CAD build for the part. Positions are in the model's coordinates, mm. A direction names the side the tool comes from. Round coordinates to 2 decimals unless told otherwise and drop trailing zeros. Loops run counter-clockwise (first coordinate to the right, second up) from the corner with the lowest first, then second, coordinate; pieces in that order, holes last.
from build123d import *

# Parameters (mm, degrees)
F0_W          = 36
F0_H          = 20
F1_DEPTH      = 3.5
F3_DEPTH      = 1
F4_W          = 4
F4_H          = 20
F4_W_2        = 8
F5_DEPTH      = 10
F6_R          = 2.5
F7_DEPTH      = 20.001
F8_R          = 5
F9_R          = 3
F10_T4_DEPTH  = 20
F10_T10_DEPTH = 20
F10_T16_DEPTH = 20
F10_T23_DEPTH = 20
F10_T29_DEPTH = 20
F10_T35_DEPTH = 20
F10_T41_DEPTH = 20
F10_T47_DEPTH = 20
F10_T54_DEPTH = 20
F10_T60_DEPTH = 20


# Not quite as in the source:
# - a fillet or chamfer that OpenCascade refuses, or shapes differently, is made with other operations: its cross-section is extruded or revolved along the edge and cut away or added


with BuildPart() as f1:
    # F0 (on Top) → F1 (new body)
    with BuildSketch(Plane.XY):
        Rectangle(F0_W, F0_H)
        with BuildLine():
            ThreePointArc((3.15, 0), (0, -3.15), (-3.15, 0))
            ThreePointArc((-3.15, 0), (0, 3.15), (3.15, 0))
        make_face(mode=Mode.SUBTRACT)
    extrude(amount=F1_DEPTH)

    # F2 (on face) → F3 (cut)
    with BuildSketch(Plane.XY.offset(3.5)):
        with BuildLine():
            Line((-1.3416407865, 2.85), (-8.05, 2.85))
            Line((-8.05, 2.85), (-8.05, -2.85))
            Line((-8.05, -2.85), (-1.3416407865, -2.85))
            ThreePointArc((-1.3416407865, -2.85), (-3.15, 0), (-1.3416407865, 2.85))
        make_face()
        with BuildLine():
            Line((1.3416407865, 2.85), (-1.3416407865, 2.85))
            ThreePointArc((-1.3416407865, 2.85), (-3.15, 0), (-1.3416407865, -2.85))
            Line((-1.3416407865, -2.85), (1.3416407865, -2.85))
            ThreePointArc((1.3416407865, -2.85), (2.6597620643, -1.6876509595), (3.15, 0))
            ThreePointArc((3.15, 0), (2.6597620643, 1.6876509595), (1.3416407865, 2.85))
        make_face()
        with BuildLine():
            Line((8.05, 2.85), (1.3416407865, 2.85))
            ThreePointArc((1.3416407865, 2.85), (2.6597620643, 1.6876509595), (3.15, 0))
            ThreePointArc((3.15, 0), (2.6597620643, -1.6876509595), (1.3416407865, -2.85))
            Line((1.3416407865, -2.85), (8.05, -2.85))
            Line((8.05, -2.85), (8.05, 2.85))
        make_face()
    extrude(amount=-F3_DEPTH, mode=Mode.SUBTRACT)

    # F4 (on Top) → F5 (join)
    with BuildSketch(Plane.XY):
        with Locations((20, 0)):
            Rectangle(F4_W, F4_H)
        with Locations((14, 0)):
            Rectangle(F4_W_2, F4_H)
        with Locations((-14, 0)):
            Rectangle(F4_W_2, F4_H)
        with Locations((-20, 0)):
            Rectangle(F4_W, F4_H)
    extrude(amount=F5_DEPTH)

    # F6 (on face) → F7 (cut, through all)
    with BuildSketch(Plane.XZ.offset(10)):
        with Locations((-16.25, 4.5)):
            Circle(F6_R)
        with BuildLine():
            ThreePointArc((18.75, 4.5), (16.25, 7), (13.75, 4.5))
            ThreePointArc((13.75, 4.5), (16.25, 2), (18.75, 4.5))
        make_face()
    extrude(amount=-F7_DEPTH, mode=Mode.SUBTRACT)

    # F8
    f8_edges = [f1.edges().sort_by_distance(p)[0] for p in [
        (-22, 0, 10),
        (-10, 0, 10),
        (10, 0, 10),
        (22, 0, 10),
    ]]
    fillet(f8_edges, radius=F8_R)

    # F9
    f9_edges = [f1.edges().sort_by_distance(p)[0] for p in [
        (-22, 0, 0),
        (22, 0, 0),
    ]]
    fillet(f9_edges, radius=F9_R)

    # F10: fillet of radius 2.5 on 2 edges, made by hand


with BuildPart() as f10_tool2:
    # F10_s3 → F10_t4 (new body)
    with BuildSketch(Plane.XZ.offset(10)):
        with BuildLine():
            ThreePointArc((10.0446437509, 5.6666666667), (9.2126670979, 4.1180683682), (7.5669656263, 3.5))
            Line((7.5669656263, 3.5), (7.5669656263, 3.25))
            Line((7.5669656263, 3.25), (10, 3.25))
            Line((10, 3.25), (10.25, 3.5))
            ThreePointArc((10.25, 3.5), (10.25, 5), (10.2924115633, 5.6333333333))
            Line((10.2924115633, 5.6333333333), (10.0446437509, 5.6666666667))
        make_face()
    extrude(amount=-F10_T4_DEPTH)

    split(bisect_by=Plane.YZ.offset(8.05), keep=Keep.TOP)

    split(bisect_by=Plane.XZ.offset(2.85), keep=Keep.TOP)


with BuildPart() as f1_1:
    add(f1.part)

    # F10_t1: union F10_tool2
    add(f10_tool2.part)


with BuildPart() as f10_tool8:
    # F10_s9 → F10_t10 (new body)
    with BuildSketch(Plane.XZ.offset(10)):
        with BuildLine():
            ThreePointArc((10.0446437509, 5.6666666667), (9.2126670979, 4.1180683682), (7.5669656263, 3.5))
            Line((7.5669656263, 3.5), (7.5669656263, 3.25))
            Line((7.5669656263, 3.25), (10, 3.25))
            Line((10, 3.25), (10.25, 3.5))
            ThreePointArc((10.25, 3.5), (10.25, 5), (10.2924115633, 5.6333333333))
            Line((10.2924115633, 5.6333333333), (10.0446437509, 5.6666666667))
        make_face()
    extrude(amount=-F10_T10_DEPTH)

    split(bisect_by=Plane.YZ.offset(8.05), keep=Keep.BOTTOM)

    split(bisect_by=Plane.XZ.offset(2.85), keep=Keep.TOP)


with BuildPart() as f1_2:
    add(f1_1.part)

    # F10_t7: union F10_tool8
    add(f10_tool8.part)


with BuildPart() as f10_tool14:
    # F10_s15 → F10_t16 (new body)
    with BuildSketch(Plane.XZ.offset(10)):
        with BuildLine():
            ThreePointArc((10.0446437509, 5.6666666667), (9.2126670979, 4.1180683682), (7.5669656263, 3.5))
            Line((7.5669656263, 3.5), (7.5669656263, 3.25))
            Line((7.5669656263, 3.25), (10, 3.25))
            Line((10, 3.25), (10.25, 3.5))
            ThreePointArc((10.25, 3.5), (10.25, 5), (10.2924115633, 5.6333333333))
            Line((10.2924115633, 5.6333333333), (10.0446437509, 5.6666666667))
        make_face()
    extrude(amount=-F10_T16_DEPTH)

    split(bisect_by=Plane.XZ.offset(-2.85), keep=Keep.TOP)

    split(bisect_by=Plane.YZ.offset(8.05), keep=Keep.TOP)

    split(bisect_by=Plane.XZ.offset(2.85), keep=Keep.BOTTOM)


with BuildPart() as f1_3:
    add(f1_2.part)

    # F10_t13: union F10_tool14
    add(f10_tool14.part)


with BuildPart() as f10_tool21:
    # F10_s22 → F10_t23 (new body)
    with BuildSketch(Plane.XZ.offset(10)):
        with BuildLine():
            ThreePointArc((10.0446437509, 5.6666666667), (9.2126670979, 4.1180683682), (7.5669656263, 3.5))
            Line((7.5669656263, 3.5), (7.5669656263, 3.25))
            Line((7.5669656263, 3.25), (10, 3.25))
            Line((10, 3.25), (10.25, 3.5))
            ThreePointArc((10.25, 3.5), (10.25, 5), (10.2924115633, 5.6333333333))
            Line((10.2924115633, 5.6333333333), (10.0446437509, 5.6666666667))
        make_face()
    extrude(amount=-F10_T23_DEPTH)

    split(bisect_by=Plane.XZ.offset(-2.85), keep=Keep.BOTTOM)

    split(bisect_by=Plane.YZ.offset(8.05), keep=Keep.TOP)


with BuildPart() as f1_4:
    add(f1_3.part)

    # F10_t20: union F10_tool21
    add(f10_tool21.part)


with BuildPart() as f10_tool27:
    # F10_s28 → F10_t29 (new body)
    with BuildSketch(Plane.XZ.offset(10)):
        with BuildLine():
            ThreePointArc((10.0446437509, 5.6666666667), (9.2126670979, 4.1180683682), (7.5669656263, 3.5))
            Line((7.5669656263, 3.5), (7.5669656263, 3.25))
            Line((7.5669656263, 3.25), (10, 3.25))
            Line((10, 3.25), (10.25, 3.5))
            ThreePointArc((10.25, 3.5), (10.25, 5), (10.2924115633, 5.6333333333))
            Line((10.2924115633, 5.6333333333), (10.0446437509, 5.6666666667))
        make_face()
    extrude(amount=-F10_T29_DEPTH)

    split(bisect_by=Plane.XZ.offset(-2.85), keep=Keep.BOTTOM)

    split(bisect_by=Plane.YZ.offset(8.05), keep=Keep.BOTTOM)


with BuildPart() as f1_5:
    add(f1_4.part)

    # F10_t26: union F10_tool27
    add(f10_tool27.part)


with BuildPart() as f10_tool33:
    # F10_s34 → F10_t35 (new body)
    with BuildSketch(Plane.XZ.offset(-10)):
        with BuildLine():
            ThreePointArc((-7.5669656263, 3.5), (-9.2126670979, 4.1180683682), (-10.0446437509, 5.6666666667))
            Line((-10.0446437509, 5.6666666667), (-10.2924115633, 5.6333333333))
            ThreePointArc((-10.2924115633, 5.6333333333), (-10.25, 5), (-10.25, 3.5))
            Line((-10.25, 3.5), (-10, 3.25))
            Line((-10, 3.25), (-7.5669656263, 3.25))
            Line((-7.5669656263, 3.25), (-7.5669656263, 3.5))
        make_face()
    extrude(amount=F10_T35_DEPTH)

    split(bisect_by=Plane.XZ.offset(-2.85), keep=Keep.BOTTOM)

    split(bisect_by=Plane.YZ.offset(-8.05), keep=Keep.TOP)


with BuildPart() as f1_6:
    add(f1_5.part)

    # F10_t32: union F10_tool33
    add(f10_tool33.part)


with BuildPart() as f10_tool39:
    # F10_s40 → F10_t41 (new body)
    with BuildSketch(Plane.XZ.offset(-10)):
        with BuildLine():
            ThreePointArc((-7.5669656263, 3.5), (-9.2126670979, 4.1180683682), (-10.0446437509, 5.6666666667))
            Line((-10.0446437509, 5.6666666667), (-10.2924115633, 5.6333333333))
            ThreePointArc((-10.2924115633, 5.6333333333), (-10.25, 5), (-10.25, 3.5))
            Line((-10.25, 3.5), (-10, 3.25))
            Line((-10, 3.25), (-7.5669656263, 3.25))
            Line((-7.5669656263, 3.25), (-7.5669656263, 3.5))
        make_face()
    extrude(amount=F10_T41_DEPTH)

    split(bisect_by=Plane.XZ.offset(-2.85), keep=Keep.BOTTOM)

    split(bisect_by=Plane.YZ.offset(-8.05), keep=Keep.BOTTOM)


with BuildPart() as f1_7:
    add(f1_6.part)

    # F10_t38: union F10_tool39
    add(f10_tool39.part)


with BuildPart() as f10_tool45:
    # F10_s46 → F10_t47 (new body)
    with BuildSketch(Plane.XZ.offset(-10)):
        with BuildLine():
            ThreePointArc((-7.5669656263, 3.5), (-9.2126670979, 4.1180683682), (-10.0446437509, 5.6666666667))
            Line((-10.0446437509, 5.6666666667), (-10.2924115633, 5.6333333333))
            ThreePointArc((-10.2924115633, 5.6333333333), (-10.25, 5), (-10.25, 3.5))
            Line((-10.25, 3.5), (-10, 3.25))
            Line((-10, 3.25), (-7.5669656263, 3.25))
            Line((-7.5669656263, 3.25), (-7.5669656263, 3.5))
        make_face()
    extrude(amount=F10_T47_DEPTH)

    split(bisect_by=Plane.XZ.offset(-2.85), keep=Keep.TOP)

    split(bisect_by=Plane.YZ.offset(-8.05), keep=Keep.BOTTOM)

    split(bisect_by=Plane.XZ.offset(2.85), keep=Keep.BOTTOM)


with BuildPart() as f1_8:
    add(f1_7.part)

    # F10_t44: union F10_tool45
    add(f10_tool45.part)


with BuildPart() as f10_tool52:
    # F10_s53 → F10_t54 (new body)
    with BuildSketch(Plane.XZ.offset(-10)):
        with BuildLine():
            ThreePointArc((-7.5669656263, 3.5), (-9.2126670979, 4.1180683682), (-10.0446437509, 5.6666666667))
            Line((-10.0446437509, 5.6666666667), (-10.2924115633, 5.6333333333))
            ThreePointArc((-10.2924115633, 5.6333333333), (-10.25, 5), (-10.25, 3.5))
            Line((-10.25, 3.5), (-10, 3.25))
            Line((-10, 3.25), (-7.5669656263, 3.25))
            Line((-7.5669656263, 3.25), (-7.5669656263, 3.5))
        make_face()
    extrude(amount=F10_T54_DEPTH)

    split(bisect_by=Plane.YZ.offset(-8.05), keep=Keep.TOP)

    split(bisect_by=Plane.XZ.offset(2.85), keep=Keep.TOP)


with BuildPart() as f1_9:
    add(f1_8.part)

    # F10_t51: union F10_tool52
    add(f10_tool52.part)


with BuildPart() as f10_tool58:
    # F10_s59 → F10_t60 (new body)
    with BuildSketch(Plane.XZ.offset(-10)):
        with BuildLine():
            ThreePointArc((-7.5669656263, 3.5), (-9.2126670979, 4.1180683682), (-10.0446437509, 5.6666666667))
            Line((-10.0446437509, 5.6666666667), (-10.2924115633, 5.6333333333))
            ThreePointArc((-10.2924115633, 5.6333333333), (-10.25, 5), (-10.25, 3.5))
            Line((-10.25, 3.5), (-10, 3.25))
            Line((-10, 3.25), (-7.5669656263, 3.25))
            Line((-7.5669656263, 3.25), (-7.5669656263, 3.5))
        make_face()
    extrude(amount=F10_T60_DEPTH)

    split(bisect_by=Plane.YZ.offset(-8.05), keep=Keep.BOTTOM)

    split(bisect_by=Plane.XZ.offset(2.85), keep=Keep.TOP)


with BuildPart() as f1_10:
    add(f1_9.part)

    # F10_t57: union F10_tool58
    add(f10_tool58.part)


solid = f1_10.part
Item 1: Mould opens along Z. For faces 1 (the cylindrical face through (-18.748, -0.14, 4.61)), 2 (the cylindrical face through (-9.19, 0.14, 4.1)), 3 (the flat face through (-4, 0, 0)) say: released by +Z, released by -Z, zero draft, split by the parting line, or undercut.
Verdict:
face 1: undercut
face 2: released by +Z
face 3: released by -Z
Item 2: Wall check: L1, parallel to X at y = -5, z = 5.25; L2, parallel to Z at x = 16.25, y = 5.5; L3, parallel to X at y = 7.25, z = 4.25. Give the ranges that are in metal, low to high.
Verdict:
L1: x = -21.99 to -18.63, -13.87 to -9.95, 9.95 to 13.87, 18.63 to 21.99
L2: z = 0 to 2, 7 to 10
L3: x = -22 to -18.74, -13.76 to -9.35, 9.35 to 13.76, 18.74 to 22
Item 3: Cut at C-C (y = 7.25). List the corners of the cut face in (x, z), plus the area to 3 significant figures.
Verdict:
outline: (-22, 3) arc R3 ccw to (-19, 0) - (19, 0) arc R3 ccw to (22, 3) - (22, 5) arc R5 ccw to (17, 10) - (15, 10) arc R5 ccw to (10.04, 5.67) arc R2.5 cw to (7.57, 3.5) - (-7.57, 3.5) arc R2.5 cw to (-10.04, 5.67) arc R5 ccw to (-15, 10) - (-17, 10) arc R5 ccw to (-22, 5) - close; hole circle Ø5 at (-16.25, 4.5); hole circle Ø5 at (16.25, 4.5)
area: 248 mm2
Item 4: Cut at A-A (x = 16.25). List the corners of the cut face in (y, z).
Verdict:
outline: (-10, 0) - (10, 0) - (10, 2) - (-10, 2) - close; (-10, 7) - (10, 7) - (10, 10) - (-10, 10) - close
Item 5: Flat gauge pins, fed straight in: P1, Ø10, axis at x = 0, y = 0, coming from the +Z side; P2, Ø3, axis at x = 3.5, y = 1, coming from the +Z side; P3, Ø2, axis at x = 11, y = -6, coming from the +Z side. Where does each tip first touch, or does it go through?
Verdict:
P1: stops at z = 3.5
P2: stops at z = 2.5
P3: stops at z = 9
Item 6: Cut at D-D (x = 0). List the corners of the cut face in (y, z), plus the area to 4 significant figures.
Verdict:
outline: (-10, 0) - (-3.15, 0) - (-3.15, 3.5) - (-10, 3.5) - close; (3.15, 0) - (10, 0) - (10, 3.5) - (3.15, 3.5) - close
area: 47.95 mm2
Item 7: 3-axis set-ups, long thin cutter, end or side, ignore diameter. For faces 4 (the cylindrical face through (12, 0, 9)), 5 (the flat face through (-5, 0, 2.5)), 6 (the cylindrical face through (21, 0, 8)): which of +Z, -Z, +X, -X, +Y, -Y reach the whole face in a straight line?
Verdict:
face 4: +Z, +Y, -Y
face 5: +Z
face 6: +Z, +X, +Y, -Y
Item 8: Cut at B-B (y = 0). List the corners of the cut face in (x, z), plus the area to 3 significant figures.
Verdict:
outline: (-22, 3) arc R3 ccw to (-19, 0) - (-3.15, 0) - (-3.15, 2.5) - (-8.05, 2.5) - (-8.05, 3.55) arc R2.5 cw to (-10.04, 5.67) arc R5 ccw to (-15, 10) - (-17, 10) arc R5 ccw to (-22, 5) - close; (3.15, 0) - (19, 0) arc R3 ccw to (22, 3) - (22, 5) arc R5 ccw to (17, 10) - (15, 10) arc R5 ccw to (10.04, 5.67) arc R2.5 cw to (8.05, 3.55) - (8.05, 2.5) - (3.15, 2.5) - close; hole circle Ø5 at (-16.25, 4.5); hole circle Ø5 at (16.25, 4.5)
area: 216 mm2
